Work out the finished part from the listing and answer in its coordinate system (mm). Face numbers are marked on the shaded views. A direction names the side the tool comes from. Give positions to 0.01 mm unless a question says otherwise; leave off trailing zeros. Order: outer loops, then holes, each group sorted by start corner. A loop starts at its lowest first (then second) coordinate and runs counter-clockwise, first axis right, second up. Notation, with made-up numbers: (24, 13.25) -> (39, 13.25) arc R9 cw to (39, 22.25) -> close; hole circle Ø1 at (-30, -8). An arc over 180 degrees is marked (long way). Use a Markdown table: item, result. Add a question column.
Autodesk Inventor part; units mm, degrees
ref_plane "YZ Plane" through (0, 0, 0) normal (1, 0, 0) x (0, 1, 0)
ref_plane "XZ Plane" through (0, 0, 0) normal (0, 1, 0) x (-1, 0, 0)
ref_plane "XY Plane" through (0, 0, 0) normal (0, 0, 1) x (1, 0, 0)
sketch "Sketch1" plane through (0, 0, 0) normal (0, 1, 0) x (-1, 0, 0)
  circle A0 centre (0, 0) radius 40
  dimension "d0" = 80
extrude "Extrusion1" add sketch "Sketch1" along normal blind 140
sketch "Sketch2" plane through (0, 140, 0) normal (0, 1, 0) x (1, 0, 0)
  line L0 (-49, -23) -> (-33, -23)
  line L1 (-33, -23) -> (-33, 22)
  line L2 (-33, 22) -> (-49, 22)
  line L3 (-49, 22) -> (-49, -23)
  point P0 (0, 0)
extrude "Extrusion2" add sketch "Sketch2" against normal blind 140
sketch "Sketch3" plane through (0, 140, 0) normal (0, 1, 0) x (1, 0, 0)
  circle A0 centre (0, 0) radius 36
  arc A1 (-33, -22.6053) -> (-33.4066, 22) centre (0, 0) ccw
  dimension "d25" = 72
extrude "Extrusion3" cut sketch "Sketch3" against normal blind 140
sketch "Sketch4" plane through (0, 140, 0) normal (0, 1, 0) x (1, 0, 0)
  line L0 (-45, 25) -> (-40.7, 25)
  line L1 (-40.7, 25) -> (-40.7, -27)
  line L2 (-40.7, -27) -> (-45, -27)
  line L3 (-45, -27) -> (-45, 25)
  line L4 (-49, 22) -> (-49, -23)
  point P0 (0, 0)
  dimension "d9" = 4.3
  dimension "d10" = 4
extrude "Extrusion4" cut sketch "Sketch4" against normal blind 50
sketch "Sketch5" plane through (0, 140, 0) normal (0, 1, 0) x (1, 0, 0)
  line L0 (37.2, -16) -> (41.5, -16)
  line L1 (41.5, -16) -> (41.5, 16)
  line L2 (41.5, 16) -> (37.2, 16)
  line L3 (37.2, 16) -> (37.2, -16)
  point P0 (0, 0)
  point P1 (39.35, -16)
  dimension "d13" = 4.3
  dimension "d14" = 32
extrude "Extrusion5" add sketch "Sketch5" against normal blind 20
sketch "Sketch6" plane through (0, 140, 0) normal (0, 1, 0) x (1, 0, 0)
  line L0 (37, 12) -> (43.2, 12)
  line L1 (43.2, 12) -> (43.2, -11)
  line L2 (43.2, -11) -> (37, -11)
  line L3 (37, -11) -> (37, 12)
  line L4 (41.5, 16) -> (37.2, 16)
  line L5 (37.2, -16) -> (41.5, -16)
  circle A0 centre (0, 0) radius 36
  point P0 (40.1, 12)
  point P1 (40.1, -11)
  dimension "d28" = 23
  dimension "d29" = 37
  dimension "d30" = 5
  dimension "d31" = 6.2
extrude "Extrusion6" cut sketch "Sketch6" against normal blind 11.8 contours L0 L1 L2 L3
properties part number "Feeder"
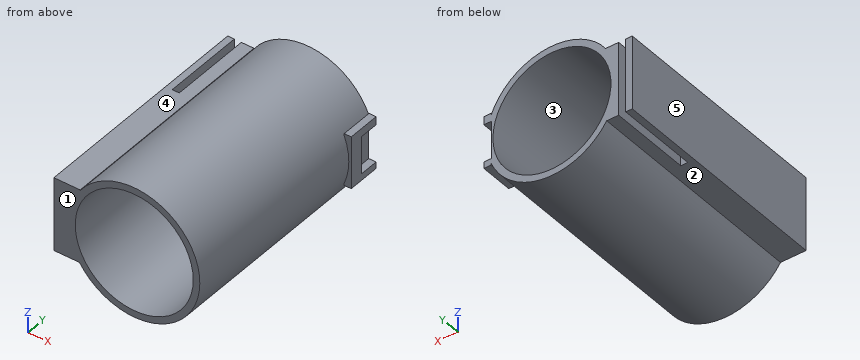
1) The part is cut by section A-A, the plane y = 124. Determine the outline of the cut face in (x, z).
2) Flat-ended cylindrical pins translate along their axes: pin 1 (5 mm diameter, centred on x = 40, y = 132, fed in from +Z); pin 2 (6 mm diameter, centred on x = -20.5, y = 119.5, fed in from +Z); pin 3 (2 mm diameter, centred on x = 39.5, z = 4.5, fed in from +Y); pin 4 (10 mm diameter, centred on y = 67, z = 26, fed in from -X). Find the tip coordinate at first contact, or state that the pin passes through.
3) Straight lines are drawn through the part: line 1 (X direction, y = 103.5, z = 0); line 2 (Z direction, x = 0, y = 51.5); line 3 (X direction, y = 93.5, z = -16). For each, find the intervals that lie inside material, in ascending order.
4) Which of the six approach directions +Z, -Z, +X, -X, +Y, -Y give full straight-line access (tool end or side, diameter ignored) to the marked faces 4 and 5?
5) The part is cut by section D-D, the plane y = 109. Determine the outline of the cut face in (x, z).
6) Determine the mould class of the marked faces 1, 2 and 3 for opening direction Z: released by +Z, released by -Z, zero draft, split by the parting line, or undercut.
7) The part is cut by section B-B, the plane x = 0. Determine the outline of the cut face in (y, z).
8) The part is cut by section C-C, the plane z = 0. Determine the outline of the cut face in (x, y).
A:
| question | item | result |
|---|---|---|
| 1 | outline | (-49, -22) -> (-45, -22) -> (-45, 23) -> (-49, 23) -> close; (-40.7, -22) -> (-33.41, -22) arc R40 ccw to (37.2, -14.7) -> (37.2, -16) -> (41.5, -16) -> (41.5, 16) -> (37.2, 16) -> (37.2, 14.7) arc R40 ccw to (-33, 22.61) -> (-33, 23) -> (-40.7, 23) -> close; hole circle Ø72 at (0, 0) |
| 2 | pin 1 | z = 16 |
| 2 | pin 2 | z = 35.97 |
| 2 | pin 3 | y = 128.2 |
| 2 | pin 4 | x = -49 |
| 3 | line 1 | -49 to -45, -40.7 to -36, 36 to 40 |
| 3 | line 2 | -40 to -36, 36 to 40 |
| 3 | line 3 | -49 to -45, -40.7 to -32.25, 32.25 to 36.66 |
| 4 | face 4 | +Z, -X, +Y, -Y |
| 4 | face 5 | +Z, -Z, -X, +Y, -Y |
| 5 | outline | (-49, -22) -> (-45, -22) -> (-45, 23) -> (-49, 23) -> close; (-40.7, -22) -> (-33.41, -22) arc R40 ccw (long way) to (-33, 22.61) -> (-33, 23) -> (-40.7, 23) -> close; hole circle Ø72 at (0, 0) |
| 6 | face 1 | zero draft |
| 6 | face 2 | released by -Z |
| 6 | face 3 | undercut |
| 7 | outline | (0, -40) -> (140, -40) -> (140, -36) -> (0, -36) -> close; (0, 36) -> (140, 36) -> (140, 40) -> (0, 40) -> close |
| 8 | outline | (-49, 0) -> (-36, 0) -> (-36, 140) -> (-40.7, 140) -> (-40.7, 90) -> (-45, 90) -> (-45, 140) -> (-49, 140) -> close; (36, 0) -> (40, 0) -> (40, 120) -> (41.5, 120) -> (41.5, 128.2) -> (37, 128.2) -> (37, 140) -> (36, 140) -> close |
